from build123d import *

# Parameters (mm, degrees)
F0_W     = 6.35
F0_H     = 31.75
F0_W_2   = 50.8
F0_H_2   = 6.35
F0_W_3   = 82.55
F0_H_3   = 12.7
F1_DEPTH = 6.35
F2_R     = 6.35
F3_R     = 25.4
F4_R     = 3.175
F6_DEPTH = 6.35
F7_R     = 1.58749
F8_SIZE  = 3.175


# Not quite as in the source:
# - a fillet or chamfer is up to 0.001 mm smaller than in the source, because OpenCascade refuses the exact size


with BuildPart() as f1:
    # F0 (on Front) → F1 (new body)
    with BuildSketch(Plane.XZ):
        Polygon((120.65, 76.2), (-127, 76.2), (-127, -76.2), (-88.9, -76.2), (25.4, 0), (120.65, 0), (120.65, 6.35), (127, 6.35), (127, 31.75), (120.65, 31.75), (120.65, 44.45), (127, 44.45), (127, 69.85), (120.65, 69.85), align=None)
        Polygon((2.5047494008, 0), (-88.9, -60.9364996005), (-88.9, 0), align=None, mode=Mode.SUBTRACT)
        with Locations((-111.125, 34.925)):
            Rectangle(F0_W, F0_H, mode=Mode.SUBTRACT)
        with Locations((-50.8, 9.525)):
            Rectangle(F0_W_2, F0_H_2, mode=Mode.SUBTRACT)
        with Locations((-60.325, 63.5)):
            Rectangle(F0_W_3, F0_H_3, mode=Mode.SUBTRACT)
        with Locations((63.5, 9.525)):
            Rectangle(F0_W_2, F0_H_2, mode=Mode.SUBTRACT)
        with Locations((60.325, 63.5)):
            Rectangle(F0_W_3, F0_H_3, mode=Mode.SUBTRACT)
    extrude(amount=F1_DEPTH)

    # F2
    f2_edges = [f1.edges().sort_by_distance(p)[0] for p in [
        (2.504749, -3.175, 0),
        (-88.9, -3.175, -60.9365),
        (-88.9, -3.175, 0),
    ]]
    fillet(f2_edges, radius=F2_R)

    # F3
    f3_edges = [f1.edges().sort_by_distance(p)[0] for p in [
        (25.4, -3.175, 0),
        (-88.9, -3.175, -76.2),
    ]]
    fillet(f3_edges, radius=F3_R)

    # F4
    f4_edges = [f1.edges().sort_by_distance(p)[0] for p in [
        (-101.6, -3.175, 57.15),
        (-101.6, -3.175, 69.85),
        (-19.05, -3.175, 57.15),
        (-19.05, -3.175, 69.85),
        (101.6, -3.175, 69.85),
        (101.6, -3.175, 57.15),
        (19.05, -3.175, 57.15),
        (19.05, -3.175, 69.85),
    ]]
    fillet(f4_edges, radius=F4_R)

    # F5 (on face) → F6 (join)
    with BuildSketch(Plane.XZ.offset(6.35)):
        Polygon((-127, 69.85), (-127, 76.2), (-133.35, 76.2), (-133.35, 63.5), (-130.175, 63.5), (-130.175, 69.85), align=None)
        Polygon((-130.175, -63.5), (-127, -63.5), (-127, -57.15), (-133.35, -57.15), (-133.35, -69.85), (-130.175, -69.85), align=None)
        Polygon((-127, -63.5), (-127, -57.15), (-133.35, -57.15), (-133.35, -69.85), (-130.175, -69.85), (-130.175, -63.5), align=None)
    extrude(amount=-F6_DEPTH)

    # F7 (radius 1.5875 in the source; OpenCascade refuses exactly that, so slightly less here)
    f7_edges = [f1.edges().sort_by_distance(p)[0] for p in [
        (-127, -3.175, 69.85),
        (-130.175, -3.175, 69.85),
        (-130.175, -3.175, -63.5),
        (-127, -3.175, -63.5),
    ]]
    fillet(f7_edges, radius=F7_R)

    # F8
    f8_edges = [f1.edges().sort_by_distance(p)[0] for p in [
        (-133.35, -3.175, 76.2),
        (-133.35, -3.175, -57.15),
    ]]
    chamfer(f8_edges, length=F8_SIZE)


solid = f1.part
Could you check a few things on this model? Use its own coordinates, in mm. A direction names the side the tool comes from. Coordinates: 2 decimals unless noted, no trailing zeros. Loops run counter-clockwise (first coordinate to the right, second up) from the corner with the lowest first, then second, coordinate; pieces in that order, holes last. Notation, with made-up numbers: (15, 52) -> (64, 52) arc R34 ccw to (64, 88) -> close; hole circle Ø11 at (71.5, 11). An arc over 180 degrees is marked (long way). Answer in a Markdown table with one row per item.
(1) If I drill on probe 1 along Z at (x, y) = (50, -2); probe 2 along X at (y, z) = (-3.25, 8.5); probe 3 along X at (y, z) = (-4.75, 66) (3 decimals), over which ranges is the centre line in solid material (lowest first)?
Results found:
| item | result |
|---|---|
| probe 1 | z = 0 to 6.35, 12.7 to 57.15, 69.85 to 76.2 |
| probe 2 | x = -127 to -76.2, -25.4 to 38.1, 88.9 to 127 |
| probe 3 | x = -133.35 to -130.175, -127 to -101.6, -19.05 to 19.05, 101.6 to 127 |
(2) Will these pins go through, and if not, where does the flat tip stop? pin 1 Ø3 at (y, z) = (-4.5, 4) entering from +X; pin 2 Ø3 at (y, z) = (-2, -8) entering from -X; pin 3 Ø10 at (x, z) = (-86.5, 30) entering from +Y; pin 4 Ø1.5 at (x, y) = (-45, -4) entering from -Z.
Results found:
| item | result |
|---|---|
| pin 1 | stops at x = 120.65 |
| pin 2 | stops at x = -127 |
| pin 3 | stops at y = 0 |
| pin 4 | stops at z = -47.43 |
(3) Imagine slicing it at B-B (z = -30). List the corners of the cut face in (x, y) for me, plus the area to 3 significant figures.
Results found:
| item | result |
|---|---|
| outline | (-127, -6.35) -> (-88.9, -6.35) -> (-88.9, 0) -> (-127, 0) -> close; (-42.5, -6.35) -> (-19.6, -6.35) -> (-19.6, 0) -> (-42.5, 0) -> close |
| area | 387 mm^2 |
(4) Imagine slicing it at A-A (x = 69). List the corners of the cut face in (y, z) for me, plus the area to 3 significant figures.
Results found:
| item | result |
|---|---|
| outline | (-6.35, 0) -> (0, 0) -> (0, 6.35) -> (-6.35, 6.35) -> close; (-6.35, 12.7) -> (0, 12.7) -> (0, 57.15) -> (-6.35, 57.15) -> close; (-6.35, 69.85) -> (0, 69.85) -> (0, 76.2) -> (-6.35, 76.2) -> close |
| area | 363 mm^2 |
(5) Imagine slicing it at C-C (y = -1.25). Give the number of separate pieces and of enclosed holes in the cut face, plus the area to 3 significant figures.
Results found:
| item | result |
|---|---|
| separate pieces | 1 |
| enclosed holes | 6 |
| area | 21,000 mm^2 |
(6) Thinking about a two-plate mould opening in X: for faces 1 (the face through (127, -3, 19)), 2 (the face through (19.05, -3, 63)), 3 (the face through (76, -3, 0)), which applies, released by +X, released by -X, zero draft, split by the parting line, or undercut?
Results found:
| item | result |
|---|---|
| face 1 | released by +X |
| face 2 | undercut |
| face 3 | zero draft |
(7) For faces 4 (the face through (120.65, -3, 3)), 5 (the face through (-61, -3, 57.15)), 6 (the face through (-34, 0, 18)), 7 (the face through (124, -3, 31.75)), which set-ups out of +Z, -Z, +X, -X, +Y, -Y let a thin tool reach every point of the face, with its end or its side?
Results found:
| item | result |
|---|---|
| face 4 | -Z, +X, +Y, -Y |
| face 5 | +Y, -Y |
| face 6 | +Z, -Z, +X, -X, +Y |
| face 7 | +X, +Y, -Y |
